```python
from build123d import *

# Parameters (mm, degrees)
SKETCH1_W           = 50.6
SKETCH1_H           = 50
BOSS_EXTRUDE1_DEPTH = 6.8
SKETCH2_W           = 6.8
SKETCH2_H           = 34
CUT_EXTRUDE1_DEPTH  = 6.8
SKETCH3_W           = 5
SKETCH3_H           = 3.55
SKETCH3_H_2         = 2.085
SKETCH3_W_2         = 11
CUT_EXTRUDE2_DEPTH  = 6.8
FILLET1_R           = 0.5


with BuildPart() as part:
    # Sketch1 → Boss-Extrude1 (new body)
    with BuildSketch(Plane.XY):
        Rectangle(SKETCH1_W, SKETCH1_H)
    extrude(amount=BOSS_EXTRUDE1_DEPTH)

    # Sketch2 → Cut-Extrude1 (cut)
    with BuildSketch(Plane.XY.offset(6.8)):
        with Locations((21.9, 0)):
            Rectangle(SKETCH2_W, SKETCH2_H)
    cut_extrude1 = extrude(amount=-CUT_EXTRUDE1_DEPTH, mode=Mode.SUBTRACT)

    # Mirror1: Cut-Extrude1 across plane
    add(cut_extrude1.mirror(Plane(origin=(0, 0, 0), x_dir=(0, 0, 1), z_dir=(1, 0, 0))), mode=Mode.SUBTRACT)

    # Sketch3 → Cut-Extrude2 (cut)
    with BuildSketch(Plane.XY.offset(6.8)):
        with Locations((0, -10)):
            Rectangle(SKETCH3_W, SKETCH3_H)
        with Locations((-5, -12.8175)):
            Rectangle(SKETCH3_W, SKETCH3_H_2)
        with Locations((-13, -10)):
            Rectangle(SKETCH3_W_2, SKETCH3_H)
        with Locations((-5, -7.1825)):
            Rectangle(SKETCH3_W, SKETCH3_H_2)
        with Locations((-5, -10)):
            Rectangle(SKETCH3_W, SKETCH3_H)
        with Locations((5, 10)):
            Rectangle(SKETCH3_W, SKETCH3_H)
        with Locations((0, 10)):
            Rectangle(SKETCH3_W, SKETCH3_H)
        with Locations((5, 7.1825)):
            Rectangle(SKETCH3_W, SKETCH3_H_2)
        with Locations((5, 12.8175)):
            Rectangle(SKETCH3_W, SKETCH3_H_2)
        with Locations((13, 10)):
            Rectangle(SKETCH3_W_2, SKETCH3_H)
    extrude(amount=-CUT_EXTRUDE2_DEPTH, mode=Mode.SUBTRACT)

    # Fillet1
    fillet1_edges = [part.edges().sort_by_distance(p)[0] for p in [
        (2.5, -8.225, 3.4),
        (2.5, -11.775, 3.4),
        (-2.5, -13.86, 3.4),
        (-7.5, -13.86, 3.4),
        (-7.5, -6.14, 3.4),
        (-2.5, -6.14, 3.4),
        (-2.5, 8.225, 3.4),
        (-2.5, 11.775, 3.4),
        (2.5, 13.86, 3.4),
        (7.5, 13.86, 3.4),
        (7.5, 6.14, 3.4),
        (2.5, 6.14, 3.4),
    ]]
    fillet(fillet1_edges, radius=FILLET1_R)


solid = part.part
```
Check sheet for the modelled part. Datum: model origin and axes. Units: mm. A direction names the side the tool comes from. Round coordinates to 2 decimals unless told otherwise and drop trailing zeros. Write each loop counter-clockwise with the first axis right and the second up, starting at its lowest first coordinate (ties: lowest second). Pieces come first, ordered by that corner, then holes. Notation, with made-up numbers: M 45.25,30 L 78.25,30 A7 cw 78.25,35 Z; hole C 30.5,67 d10. An arc over 180 degrees is marked long. Write item = value, one per line. Start each with the question number.
1. Tool access check on faces 1 (the flat face through (25.3, -21, 3)), 2 (the flat face through (-13, -11.775, 3)), 3 (the flat face through (22, -17, 3)), 4 (the flat face through (0, -25, 3)), 5 (the flat face through (-7.5, -13, 3)). Record the directions out of +Z, -Z, +X, -X, +Y, -Y that give a thin tool (end or side, any length) a straight path to the whole face; none if there is none.
2. Scan lines: line 1 (Y direction, x = -1.5, z = 6.25) (3 decimals); line 2 (Y direction, x = 20.5, z = 4); line 3 (Y direction, x = 8.5, z = 2.5) (3 decimals). Record each from-to range of solid material in increasing order. Write a range as [from, to].
3. Section check A-A, the plane x = -1. Record the cut outline in (y, z) (3 decimals), then the cut area to 3 significant figures.
4. Section check C-C, the plane y = 2. Record the cut outline in (x, z).
5. Section check B-B, the plane x = -16. Record the cut outline in (y, z) (3 decimals).
6. Section check D-D, the plane y = 10. Record the cut outline in (x, z).
7. Gauge pin test, flat ends, axial feed: pin 1 (1.3 mm diameter, centred on y = 12.5, z = 1.5, fed in from +X); pin 2 (4 mm diameter, centred on y = -14.5, z = 3, fed in from -X). Record the tip position at first contact, or that the pin passes through.
Results found:
q1.face_1 = +Z, -Z, +X, +Y, -Y
q1.face_2 = +Z, -Z, -X
q1.face_3 = +Z, -Z, +X
q1.face_4 = +Z, -Z, +X, -X, -Y
q1.face_5 = +Z, -Z
q2.line_1 = [-25, -11.775], [-8.225, 8.225], [11.775, 25]
q2.line_2 = [-25, -17], [17, 25]
q2.line_3 = [-25, 8.225], [11.775, 25]
q3.outline = M -25,0 L -11.775,0 L -11.775,6.8 L -25,6.8 Z; M -8.225,0 L 8.225,0 L 8.225,6.8 L -8.225,6.8 Z; M 11.775,0 L 25,0 L 25,6.8 L 11.775,6.8 Z
q3.area = 292 mm^2
q4.outline = M -18.5,0 L 18.5,0 L 18.5,6.8 L -18.5,6.8 Z
q5.outline = M -25,0 L -11.775,0 L -11.775,6.8 L -25,6.8 Z; M -8.225,0 L 25,0 L 25,6.8 L -8.225,6.8 Z
q6.outline = M -18.5,0 L -2.5,0 L -2.5,6.8 L -18.5,6.8 Z
q7.pin_1 = 18.5
q7.pin_2 = -18.5
